from build123d import *

# Parameters (mm, degrees)
SKETCH_3_R          = 32.5
EXTRUDE_3_DEPTH     = 20
SKETCH_4_W          = 17.889883514
SKETCH_4_H          = 45.147936345
SKETCH_4_W_2        = 17.954509811
CUT_EXTRUDE_1_DEPTH = 40
SKETCH_5_R          = 3
CUT_EXTRUDE_2_DEPTH = 60


with BuildPart() as part:
    # Эскиз3 → Вытянуть3 (new body)
    with BuildSketch(Plane.XY):
        Circle(SKETCH_3_R)
    extrude(amount=EXTRUDE_3_DEPTH)

    # Эскиз4 → Вырез-Вытянуть1 (cut, symmetric)
    with BuildSketch(Plane(origin=(0, 0, 0), x_dir=(1, 0, 0), z_dir=(0, 1, 0))):
        with Locations((-35.944941757, -4.95296847)):
            Rectangle(SKETCH_4_W, SKETCH_4_H)
        with Locations((35.977254906, -4.95296847)):
            Rectangle(SKETCH_4_W_2, SKETCH_4_H)
    extrude(amount=CUT_EXTRUDE_1_DEPTH, both=True, mode=Mode.SUBTRACT)

    # Эскиз5 → Вырез-Вытянуть2 (cut)
    with BuildSketch(Plane(origin=(27, 0, 0), x_dir=(0, 0, -1), z_dir=(1, 0, 0))):
        with Locations((-10, 0)):
            Circle(SKETCH_5_R)
    extrude(amount=-CUT_EXTRUDE_2_DEPTH, mode=Mode.SUBTRACT)


solid = part.part
For this review, take the finished solid that the model builds, in its own axes (mm). Give positions to 0.01 mm unless a question says otherwise; leave off trailing zeros. Loops run counter-clockwise (first coordinate to the right, second up) from the corner with the lowest first, then second, coordinate; pieces in that order, holes last. Notation, with made-up numbers: (58, 8) -> (86, 8) arc R18 cw to (86, 30) -> close; hole circle Ø5 at (-20.5, 85). An arc over 180 degrees is marked (long way). One line per question, with ' | ' between items.
1) We need section D-D (z = 16.25). Write out the cut boundary in (x, y).
Resolved:
outline: (-27, -18.09) arc R32.5 ccw to (27, -18.09) -> (27, 18.09) arc R32.5 ccw to (-27, 18.09) -> close
2) The part is to be moulded in two halves that separate along Z. For faces 1 (the cylindrical face through (0.446, 32.497, 9.86)), 2 (the cylindrical face through (0.4, -1.8, 12.4)), 3 (the flat face through (0, 0, 20)), 4 (the flat face through (0, 0, 0)), say which applies: +Z half, -Z half, draft (parallel to the pull), parting line (faces both ways), or undercut.
Resolved:
face 1: draft | face 2: undercut | face 3: +Z half | face 4: -Z half
3) We need section A-A (z = 10). Write out the cut boundary in (x, y), plus the area to 3 significant figures.
Resolved:
outline: (-27, -18.09) arc R32.5 ccw to (27, -18.09) -> (27, -3) -> (-27, -3) -> close; (-27, 3) -> (27, 3) -> (27, 18.09) arc R32.5 ccw to (-27, 18.09) -> close | area: 2,720 mm2
4) To check wall thickness, follow probe 1 along Y at (x, z) = (-16, 10); probe 2 along X at (y, z) = (27, 1.25); probe 3 along Z at (x, y) = (2, -2). State the ranges of each line that lie inside material, in increasing order.
Resolved:
probe 1: y = -28.29 to -3, 3 to 28.29 | probe 2: x = -18.09 to 18.09 | probe 3: z = 0 to 7.76, 12.24 to 20
5) Insertion check: pin 1 Ø8 at (x, y) = (13, -4) entering from -Z. The pin has a flat end and moves straight along its axis. Give the tip position at first contact, or say it passes through.
Resolved:
pin 1: stops at z = 0
6) We need section B-B (y = 0). Write out the cut boundary in (x, z), plus the area to 3 significant figures.
Resolved:
outline: (-27, 0) -> (27, 0) -> (27, 7) -> (-27, 7) -> close; (-27, 13) -> (27, 13) -> (27, 20) -> (-27, 20) -> close | area: 756 mm2
7) We need section C-C (x = 16.5). Write out the cut boundary in (y, z), plus the area to 3 significant figures.
Resolved:
outline: (-28, 0) -> (28, 0) -> (28, 20) -> (-28, 20) -> close; hole circle Ø6 at (0, 10) | area: 1,090 mm2
